The figure shows three views and two pictorial views of one solid part (mm, origin at its lowest corner). Answer the questions. Give positions to 0.01 mm unless a question says otherwise; leave off trailing zeros. Order: outer loops, then holes, each group sorted by start corner. A loop starts at its lowest first (then second) coordinate and runs counter-clockwise, first axis right, second up. Notation, with made-up numbers: (41, 56) - (90, 56) arc R32 cw to (90, 84) - close; hole circle Ø7 at (41, 59). An arc over 180 degrees is marked (long way). Answer as CSV lines item,"result". Start each with the question number.
1. Section C-C on y = 182 is taken. Give the vertices of the cut face in (x, z), and give its area (3 significant figures).
2. Section A-A on y = 139 is taken. Give the vertices of the cut face in (x, z).
3. Consider line 1 along Y through (x, z) = (150, 3.2); line 2 along X through (y, z) = (138.5, 4.65); line 3 along X through (y, z) = (141, 1.1). Determine where each line is inside the solid, lowest interval first. Write a range as [from, to].
4. Section B-B on x = 150 is taken. Give the vertices of the cut face in (y, z), and give its area (3 significant figures).
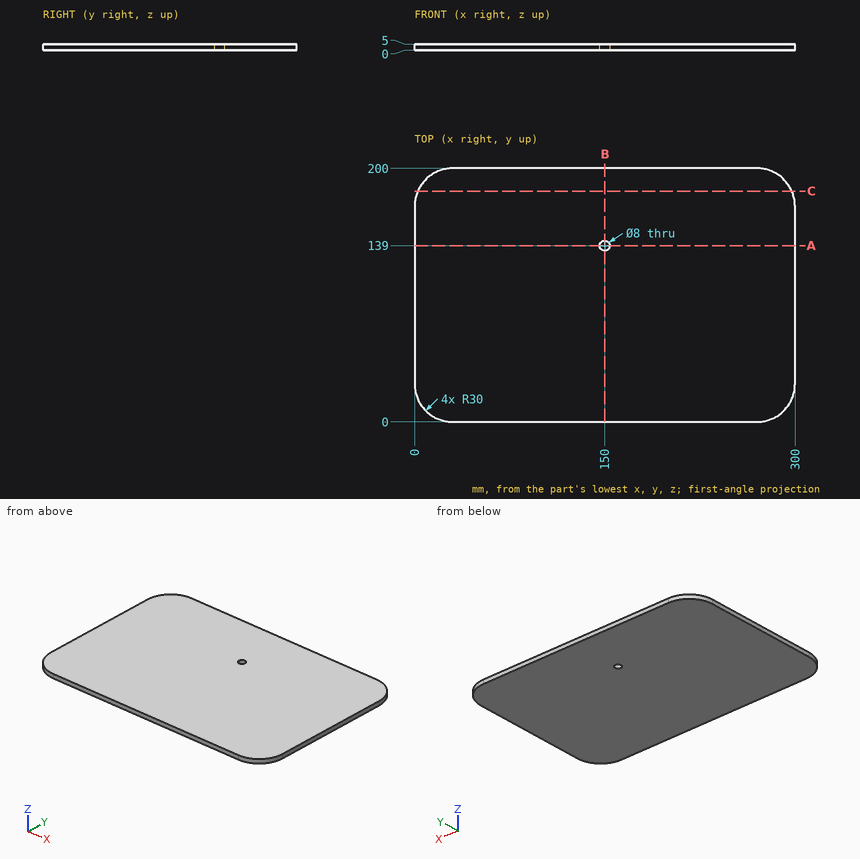
Checks:
1,outline,"(2.5, 0) - (297.5, 0) - (297.5, 5) - (2.5, 5) - close"
1,area,"1,470 mm²"
2,outline,"(0, 0) - (146, 0) - (146, 5) - (0, 5) - close; (154, 0) - (300, 0) - (300, 5) - (154, 5) - close"
3,line 1,"y = [0, 135], [143, 200]"
3,line 2,"x = [0, 146.03], [153.97, 300]"
3,line 3,"x = [0, 146.54], [153.46, 300]"
4,outline,"(0, 0) - (135, 0) - (135, 5) - (0, 5) - close; (143, 0) - (200, 0) - (200, 5) - (143, 5) - close"
4,area,"960 mm²"
